Check sheet for the modelled part. Datum: model origin and axes. Units: mm. A direction names the side the tool comes from. Give positions to 0.01 mm unless a question says otherwise; leave off trailing zeros. Loops run counter-clockwise (first coordinate to the right, second up) from the corner with the lowest first, then second, coordinate; pieces in that order, holes last.
```python
from build123d import *

# Parameters (mm, degrees)
FILLET_1_R               = 1
SKETCH_2_R               = 7.321356554
SKETCH_2_W               = 1
SKETCH_2_H               = 8.939101976
SKETCH_2_H_2             = 8.847887315
CUT_EXTRUDE_1_DEPTH      = 8
FILLET_2_R               = 0.2
CUT_EXTRUDE_2_DEPTH      = 36.355339178
CUT_EXTRUDE_2_DEPTH_BACK = 36.355339178
SKETCH_3_R               = 1.5


with BuildPart() as part:
    # 草图1 → 旋转1 (revolve)
    with BuildSketch(Plane.XY):
        Polygon((0, 0), (0, 2.25), (-22, 2.25), (-22, 3), (-27, 3), (-27, 2.5), (-35, 2.5), (-35, 0), align=None)
    revolve(axis=Axis((0, 0, 0), (-1, 0, 0)))

    # 圆角1
    fillet_1_edges = [part.edges().sort_by_distance(p)[0] for p in [
        (-35, -2.5, 0),
    ]]
    fillet(fillet_1_edges, radius=FILLET_1_R)

    # 草图2 → 切除-拉伸1 (cut)
    with BuildSketch(Plane.ZY.offset(35)):
        Circle(SKETCH_2_R)
        with Locations((-1.5, 0.70306053)):
            Rectangle(SKETCH_2_W, SKETCH_2_H, mode=Mode.SUBTRACT)
        with Locations((1.5, 0.129971064)):
            Rectangle(SKETCH_2_W, SKETCH_2_H_2, mode=Mode.SUBTRACT)
    extrude(amount=-CUT_EXTRUDE_1_DEPTH, mode=Mode.SUBTRACT)

    # 圆角2
    fillet_2_edges = [part.edges().sort_by_distance(p)[0] for p in [
        (-27, -3, 0),
        (-22, -3, 0),
        (0, -2.25, 0),
    ]]
    fillet(fillet_2_edges, radius=FILLET_2_R)

    # 草图3 → 切除-拉伸2 (cut, two sides: drawn at the far end of the back side and taken through both)
    with BuildSketch(Plane(origin=(0, 0, -1), x_dir=(-1, 0, 0), z_dir=(0, 0, -1)).offset(-CUT_EXTRUDE_2_DEPTH_BACK)):
        with Locations(Location((31.5, 0, 0), (0, 0, 270))):
            Circle(SKETCH_3_R)
    extrude(amount=CUT_EXTRUDE_2_DEPTH + CUT_EXTRUDE_2_DEPTH_BACK, mode=Mode.SUBTRACT)


solid = part.part
```
(1) Section check C-C on x = -32. Record the boundary of the cut face in (y, z), plus the area to 3 significant figures.
(2) Section check A-A on y = 0. Give the number of separate pieces and of enclosed holes in the cut face, plus the area to 3 significant figures.
(3) Release check for a two-part mould opening along Z. For faces 1 (the face through (-25, -3, 0)), 2 (the face through (-30, 1, -1)), 3 (the face through (-29, 0, 2)) record: pulls with the +Z half, pulls with the -Z half, needs draft (parallel to the pull), parting line crosses it, or undercut.
(4) Section check B-B on z = 0. Record the boundary of the cut face in (x, y), plus the area to 3 significant figures.
(5) Material ranges on line 1 (X direction, y = 0, z = 1.55); line 2 (Y direction, x = -31.5, z = 1.5); line 3 (Z direction, x = -28, y = 0.5), recorded low to high.
(6) Section check D-D on x = -3. Record the boundary of the cut face in (y, z).
(7) Access from +Z, -Z, +X, -X, +Y, -Y to the whole of each face (thin tool, end or side, straight path). Record for faces 4 (the face through (-11.25, -0.29, -2.23)), 5 (the face through (-30.5, 2, -1.5)), 6 (the face through (-30, 1, 1)).
(8) Gauge pin test, flat ends, axial feed: pin 1 Ø3.5 at (x, y) = (-33, 1) entering from +Z; pin 2 Ø3.5 at (x, y) = (-33, 0.5) entering from -Z; pin 3 Ø1.5 at (x, z) = (-26.5, -1.5) entering from +Y. Record the tip position at first contact, or that the pin passes through.
Computed values:
1. outline: (-2.29, -1) arc R2.5 ccw to (-1.5, -2) - (-1.41, -2) - (-1.41, -1) - close; (-2.29, 1) - (-1.41, 1) - (-1.41, 2) - (-1.5, 2) arc R2.5 ccw to start; (1.41, -2) - (1.5, -2) arc R2.5 ccw to (2.29, -1) - (1.41, -1) - close; (1.41, 1) - (2.29, 1) arc R2.5 ccw to (1.5, 2) - (1.41, 2) - close
1. area: 2.21 mm2
2. separate pieces: 3
2. enclosed holes: 0
2. area: 139 mm2
3. face 1: parting line crosses it
3. face 2: undercut
3. face 3: pulls with the +Z half
4. outline: (-27, -2.8) arc R0.2 ccw to (-26.8, -3) - (-22.2, -3) arc R0.2 ccw to (-22, -2.8) - (-22, -2.25) - (-0.2, -2.25) arc R0.2 ccw to (0, -2.05) - (0, 2.05) arc R0.2 ccw to (-0.2, 2.25) - (-22, 2.25) - (-22, 2.8) arc R0.2 ccw to (-22.2, 3) - (-26.8, 3) arc R0.2 ccw to (-27, 2.8) - close
4. area: 129 mm2
5. line 1: x = -35 to -33, -30 to 0
5. line 2: y = -2 to -1.5, 1.5 to 2
5. line 3: z = -2 to -1, 1 to 2
6. outline: circle Ø4.5 at (0, 0)
7. face 4: +X
7. face 5: -Z, -X, +Y
7. face 6: -X, +Y, -Y
8. pin 1: stops at z = 2
8. pin 2: stops at z = -2
8. pin 3: stops at y = 2.9
